Verification items for the finished model (mm, model axes). A direction names the side the tool comes from. Round coordinates to 2 decimals unless told otherwise and drop trailing zeros. Loops run counter-clockwise (first coordinate to the right, second up) from the corner with the lowest first, then second, coordinate; pieces in that order, holes last. Notation, with made-up numbers: M 71.25,42 L 109.25,42 A21 cw 109.25,58 Z; hole C 56,-11.75 d10. An arc over 180 degrees is marked long. One line per item, written item: value.
Autodesk Fusion 360 part; units mm, degrees
sketch "Sketch1" plane through (0, 0, 0) normal (0, 0, 1) x (1, 0, 0)
  line L0 (27.3, 35.75) -> (-27.3, 35.75)
  line L1 (-27.3, 35.75) -> (-27.3, -35.75)
  line L2 (-27.3, -35.75) -> (27.3, -35.75)
  line L3 (27.3, -35.75) -> (27.3, 35.75)
  line L4 (27.3, 35.75) -> (-27.3, -35.75) construction
  line L5 (-27.3, 35.75) -> (27.3, -35.75) construction
  dimension "d1" = 54.6
  dimension "d2" = 71.5
extrude "Extrude1" add sketch "Sketch1" along normal blind 40
sketch "Sketch2" plane through (0, 0, 40) normal (0, 0, 1) x (-1, 0, 0)
  line L0 (-27.3, 35.75) -> (-27.3, -35.75)
  line L1 (-27.3, -35.75) -> (27.3, -35.75)
  line L2 (27.3, -35.75) -> (27.3, 35.75)
  line L3 (27.3, 35.75) -> (-27.3, 35.75)
  line L4 (-25.3, -33.75) -> (25.3, -33.75)
  line L5 (25.3, -33.75) -> (25.3, 33.75)
  line L6 (25.3, 33.75) -> (-25.3, 33.75)
  line L7 (-25.3, 33.75) -> (-25.3, -33.75)
  line L8 (-25.3, -33.75) -> (25.3, 33.75) construction
  line L9 (25.3, -33.75) -> (-25.3, 33.75) construction
  dimension "d5" = 50.6
  dimension "d6" = 67.5
extrude "Extrude2" cut sketch "Sketch2" against normal blind 38 contours L4 L5 L6 L7
sketch "Sketch3" plane through (0, 0, 2) normal (0, 0, 1) x (-1, 0, 0)
  line L0 (-25.3, 33.75) -> (-25.3, -33.75)
  line L1 (-25.3, -33.75) -> (25.3, -33.75)
  line L2 (25.3, -33.75) -> (25.3, 33.75)
  line L3 (25.3, 33.75) -> (-25.3, 33.75)
  line L4 (20, 20) -> (14, 20)
  line L5 (14, 20) -> (14, 30.3)
  line L6 (14, 30.3) -> (20, 30.3)
  line L7 (20, 30.3) -> (20, 20)
  dimension "d9" = 6
  dimension "d10" = 10.3
extrude "Extrude3" cut sketch "Sketch3" against normal blind 2 contours L4 L5 L6 L7
(1) Depth check by flat-ended pin: pin 1 Ø6 at (x, y) = (7, -24) entering from -Z. Enter the tip coordinate at first touch or a pass-through.
Completed:
pin 1: stops at z = 0
(2) Thickness scan on L1, parallel to Y at x = -8, z = 14; L2, parallel to X at y = -15, z = 14.5; L3, parallel to Z at x = 5, y = 14. Record the ranges inside material, lowest first. Write a range as from..to.
Completed:
L1: y = -35.75..-33.75, 33.75..35.75
L2: x = -27.3..-25.3, 25.3..27.3
L3: z = 0..2
(3) Tool access check on faces 1 (the face through (0, 33.75, 21)), 2 (the face through (-17, -20, 1)), 3 (the face through (0, 1, 0)). Record the directions out of +Z, -Z, +X, -X, +Y, -Y that give a thin tool (end or side, any length) a straight path to the whole face; none if there is none.
Completed:
face 1: +Z
face 2: +Z, -Z
face 3: -Z, +X, -X, +Y, -Y
(4) Mould release check, pull along Y, two halves, no side actions. Record for faces 4 (the face through (-17, -30.3, 1)), 5 (the face through (0, 35.75, 20)), 6 (the face through (-27.3, 1, 20)): +Y half, -Y half, draft (parallel to the pull), parting line (faces both ways), or undercut.
Completed:
face 4: undercut
face 5: +Y half
face 6: draft
(5) Sectioned sample at B-B on x = 22.5. Enter the section's corners in (y, z).
Completed:
outline: M -35.75,0 L 35.75,0 L 35.75,40 L 33.75,40 L 33.75,2 L -33.75,2 L -33.75,40 L -35.75,40 Z
(6) Sectioned sample at D-D on y = 3.5. Enter the section's corners in (x, z), and give its area (3 significant figures).
Completed:
outline: M -27.3,0 L 27.3,0 L 27.3,40 L 25.3,40 L 25.3,2 L -25.3,2 L -25.3,40 L -27.3,40 Z
area: 261 mm^2
(7) Sectioned sample at A-A on x = -15. Enter the section's corners in (y, z), and give its area (3 significant figures).
Completed:
outline: M -35.75,0 L -30.3,0 L -30.3,2 L -33.75,2 L -33.75,40 L -35.75,40 Z; M -20,0 L 35.75,0 L 35.75,40 L 33.75,40 L 33.75,2 L -20,2 Z
area: 274 mm^2
(8) Sectioned sample at C-C on z = 14. Enter the section's corners in (x, y).
Completed:
outline: M -27.3,-35.75 L 27.3,-35.75 L 27.3,35.75 L -27.3,35.75 Z; hole M -25.3,-33.75 L 25.3,-33.75 L 25.3,33.75 L -25.3,33.75 Z
